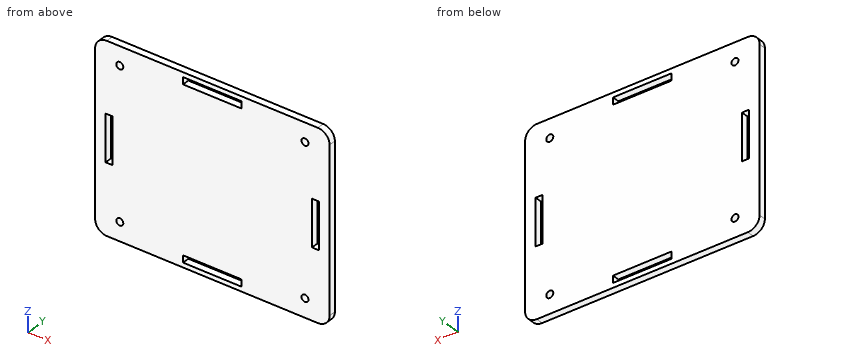
```python
from build123d import *

# Parameters (mm, degrees)
SKETCH1_W           = 100
SKETCH1_H           = 80
BOSS_EXTRUDE1_DEPTH = 3
FILLET1_R           = 5
SKETCH2_R           = 1.5
CUT_EXTRUDE1_DEPTH  = 3
SKETCH3_W           = 25
SKETCH3_H           = 3
SKETCH3_W_2         = 3
SKETCH3_H_2         = 20
CUT_EXTRUDE2_DEPTH  = 10


with BuildPart() as part:
    # Sketch1 → Boss-Extrude1 (new body)
    with BuildSketch(Plane(origin=(0, 0, 0), x_dir=(1, 0, 0), z_dir=(0, 1, 0))):
        Rectangle(SKETCH1_W, SKETCH1_H)
    extrude(amount=BOSS_EXTRUDE1_DEPTH)

    # Fillet1
    fillet1_edges = [part.edges().sort_by_distance(p)[0] for p in [
        (50, 1.5, 40),
        (-50, 1.5, 40),
        (-50, 1.5, -40),
        (50, 1.5, -40),
    ]]
    fillet(fillet1_edges, radius=FILLET1_R)

    # Sketch2 → Cut-Extrude1 (cut)
    with BuildSketch(Plane(origin=(0, 3, 0), x_dir=(1, 0, 0), z_dir=(0, 1, 0))):
        with Locations(Location((39.5, -32, 0), (0, 0, 270))):
            Circle(SKETCH2_R)
        with Locations(Location((39.5, 32, 0), (0, 0, 270))):
            Circle(SKETCH2_R)
        with Locations(Location((-39.5, 32, 0), (0, 0, 270))):
            Circle(SKETCH2_R)
        with Locations(Location((-39.5, -32, 0), (0, 0, 270))):
            Circle(SKETCH2_R)
    extrude(amount=-CUT_EXTRUDE1_DEPTH, mode=Mode.SUBTRACT)

    # Sketch3 → Cut-Extrude2 (cut)
    with BuildSketch(Plane(origin=(0, 3, 0), x_dir=(1, 0, 0), z_dir=(0, 1, 0))):
        with Locations((0, -36.5)):
            Rectangle(SKETCH3_W, SKETCH3_H)
        with Locations((0, 36.5)):
            Rectangle(SKETCH3_W, SKETCH3_H)
        with Locations((44, 0)):
            Rectangle(SKETCH3_W_2, SKETCH3_H_2)
        with Locations((-44, 0)):
            Rectangle(SKETCH3_W_2, SKETCH3_H_2)
    extrude(amount=-CUT_EXTRUDE2_DEPTH, mode=Mode.SUBTRACT)


solid = part.part
```
Read the model definition and answer for the solid it produces. Units are mm, in the model's axes. Give positions to 0.01 mm unless a question says otherwise; leave off trailing zeros. Write each loop counter-clockwise with the first axis right and the second up, starting at its lowest first coordinate (ties: lowest second). Pieces come first, ordered by that corner, then holes. Notation, with made-up numbers: M -14.5,-30.75 L -3.5,-30.75 A24 ccw -3.5,-1.75 Z; hole C -21.5,-17.5 d3. An arc over 180 degrees is marked long. Put each result on its own line as item: value. Start each with the question number.
1. Consider line 1 along X through (y, z) = (0.45, -8); line 2 along X through (y, z) = (1.9, -32); line 3 along Z through (x, y) = (-40, 2). Determine where each line is inside the solid, lowest interval first.
2. The part is cut by section C-C, the plane y = 2.2. Give the number of separate pieces and of enclosed holes in the cut face, and give its area (3 significant figures).
3. The part is cut by section B-B, the plane x = -9. Give the vertices of the cut face in (y, z), and give its area (3 significant figures).
4. This flat-tipped pin is pushed along its axis until it touches: pin 1 Ø1.5 at (y, z) = (1.5, 37) entering from -X. Where does it stop, or does it pass through?
5. The part is cut by section A-A, the plane z = -32. Give the vertices of the cut face in (x, y).
Final values:
1. line 1: x = -50 to -45.5, -42.5 to 42.5, 45.5 to 50
1. line 2: x = -50 to -41, -38 to 38, 41 to 50
1. line 3: z = -40 to -33.41, -30.59 to 30.59, 33.41 to 40
2. separate pieces: 1
2. enclosed holes: 8
2. area: 7,680 mm²
3. outline: M 0,-40 L 3,-40 L 3,-38 L 0,-38 Z; M 0,-35 L 3,-35 L 3,35 L 0,35 Z; M 0,38 L 3,38 L 3,40 L 0,40 Z
3. area: 222 mm²
4. pin 1: stops at x = -49.84
5. outline: M -50,0 L -41,0 L -41,3 L -50,3 Z; M -38,0 L 38,0 L 38,3 L -38,3 Z; M 41,0 L 50,0 L 50,3 L 41,3 Z
